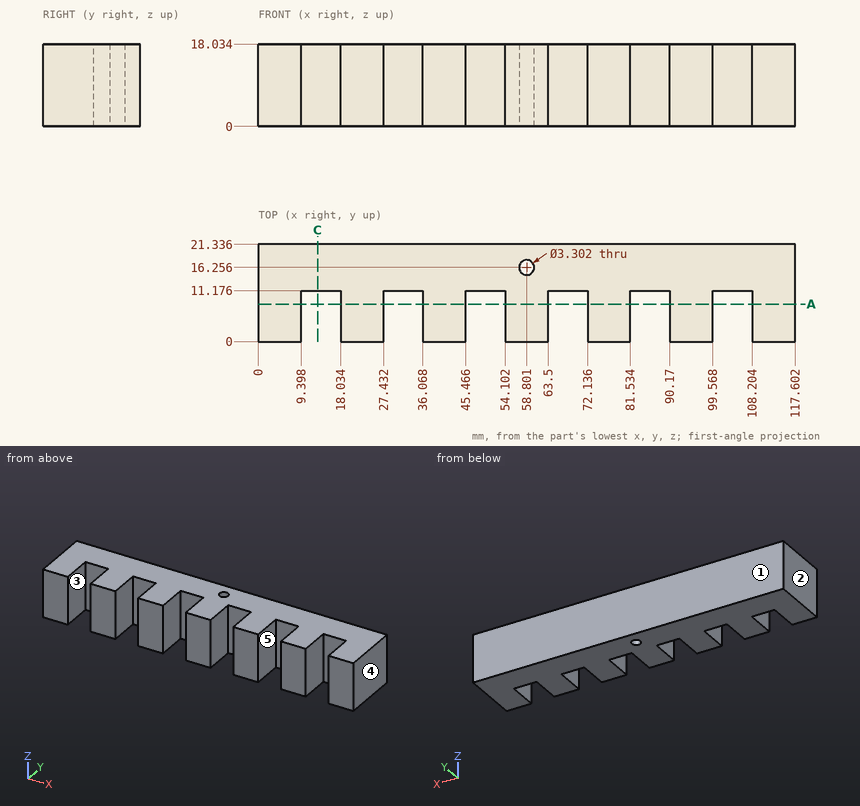
Source: three-view drawing plus pictorial views. Frame: mm from the lowest corner of the part. A direction names the side the tool comes from. Round coordinates to 2 decimals unless told otherwise and drop trailing zeros. Write each loop counter-clockwise with the first axis right and the second up, starting at its lowest first coordinate (ties: lowest second). Pieces come first, ordered by that corner, then holes. Notation, with made-up numbers: M 45.5,74 L 101.5,74 A19 cw 101.5,102 Z; hole C -11.5,-22 d9. An arc over 180 degrees is marked long. Write each question's results on one line, items separated by ' | '.
Q1. Section query A-A (y = 8.25). Return loops of the section in (x, z), and give its area (3 significant figures).
Results:
outline: M 0,0 L 9.4,0 L 9.4,18.03 L 0,18.03 Z; M 18.03,0 L 27.43,0 L 27.43,18.03 L 18.03,18.03 Z; M 36.07,0 L 45.47,0 L 45.47,18.03 L 36.07,18.03 Z; M 54.1,0 L 63.5,0 L 63.5,18.03 L 54.1,18.03 Z; M 72.14,0 L 81.53,0 L 81.53,18.03 L 72.14,18.03 Z; M 90.17,0 L 99.57,0 L 99.57,18.03 L 90.17,18.03 Z; M 108.2,0 L 117.6,0 L 117.6,18.03 L 108.2,18.03 Z | area: 1,190 mm^2
Q2. Pin query (flat end, axial travel): P1, Ø4.5, axis at x = 86, z = 7, coming from the -Y side; P2, Ø3, axis at x = 58.801, y = 16.256, coming from the -Z side. Return the tip coordinate at first contact, or that it passes through.
Results:
P1: stops at y = 11.18 | P2: passes through
Q3. Access query for the marked faces 4 and 5. Directions: +Z, -Z, +X, -X, +Y, -Y. A direction counts if a zero-diameter tool reaches every point of the face in a straight line with its end or side. Return the directions, or none.
Results:
face 4: +Z, -Z, +X, +Y, -Y | face 5: +Z, -Z, -Y
Q4. Line query: line 1 along Y through (x, z) = (32, 3); line 2 along X through (y, z) = (15.75, 15); line 3 along Y through (x, z) = (57.5, 14.5). Output: solid intervals per line, ascending.
Results:
line 1: y = 11.18 to 21.34 | line 2: x = 0 to 57.23, 60.37 to 117.6 | line 3: y = 0 to 15.24, 17.27 to 21.34
Q5. Draft query along X for the marked faces 1, 2 and 3. Return one class per face: released by +X, released by -X, zero draft, split by the parting line, or undercut.
Results:
face 1: zero draft | face 2: released by -X | face 3: undercut
Q6. Section query C-C (x = 13). Return loops of the section in (y, z), and give its area (3 significant figures).
Results:
outline: M 11.18,0 L 21.34,0 L 21.34,18.03 L 11.18,18.03 Z | area: 183 mm^2
